```python
from build123d import *

# Parameters (mm, degrees)
SKETCH1_W                = 25
SKETCH1_H                = 25
SKETCH1_W_2              = 21
SKETCH1_H_2              = 21
BOSS_EXTRUDE1_DEPTH      = 200
SKETCH2_W                = 40
SKETCH2_H                = 12
CUT_EXTRUDE1_DEPTH       = 26
SKETCH3_R                = 5
CUT_EXTRUDE2_DEPTH       = 26
BOSS_EXTRUDE2_START      = -40
SKETCH5_W                = 21
SKETCH5_H                = 21
BOSS_EXTRUDE2_DEPTH      = 1
BOSS_EXTRUDE2_DEPTH_BACK = 199
SKETCH3_2_R              = 5
CUT_EXTRUDE4_DEPTH       = 239
SKETCH6_W                = 21
SKETCH6_H                = 12
CUT_EXTRUDE5_DEPTH       = 39
SKETCH8_W                = 21
SKETCH8_H                = 12
BOSS_EXTRUDE3_DEPTH      = 40
SKETCH9_R                = 5
CUT_EXTRUDE6_DEPTH       = 19.5


with BuildPart() as part:
    # Sketch1 → Boss-Extrude1 (new body)
    with BuildSketch(Plane.XY):
        Rectangle(SKETCH1_W, SKETCH1_H)
        Rectangle(SKETCH1_W_2, SKETCH1_H_2, mode=Mode.SUBTRACT)
    extrude(amount=BOSS_EXTRUDE1_DEPTH)

    # Sketch2 → Cut-Extrude1 (cut, through all)
    with BuildSketch(Plane(origin=(12.5, 0, 0), x_dir=(0, 0, -1), z_dir=(1, 0, 0))):
        with Locations((-20, 0)):
            Rectangle(SKETCH2_W, SKETCH2_H)
    extrude(amount=-CUT_EXTRUDE1_DEPTH, mode=Mode.SUBTRACT)

    # Sketch3 → Cut-Extrude2 (cut, through all)
    with BuildSketch(Plane(origin=(0, 12.5, 0), x_dir=(1, 0, 0), z_dir=(0, 1, 0))):
        with Locations((0, -9)):
            Circle(SKETCH3_R)
    extrude(amount=-CUT_EXTRUDE2_DEPTH, mode=Mode.SUBTRACT)

    # Sketch5 → Boss-Extrude2 (add, two sides)
    with BuildSketch(Plane.XY.offset(240).offset(BOSS_EXTRUDE2_START)) as boss_extrude2_sk:
        Rectangle(SKETCH5_W, SKETCH5_H)
    extrude(amount=BOSS_EXTRUDE2_DEPTH)
    extrude(boss_extrude2_sk.sketch, amount=-BOSS_EXTRUDE2_DEPTH_BACK)

    # Sketch3<2> → Cut-Extrude4 (cut)
    with BuildSketch(Plane(origin=(0, 12.5, 0), x_dir=(1, 0, 0), z_dir=(0, 1, 0))):
        with Locations((0, -9)):
            Circle(SKETCH3_2_R)
    extrude(amount=-CUT_EXTRUDE4_DEPTH, mode=Mode.SUBTRACT)

    # Sketch6 → Cut-Extrude5 (cut)
    with BuildSketch(Plane(origin=(0, 0, 1), x_dir=(-1, 0, 0), z_dir=(0, 0, -1))):
        Rectangle(SKETCH6_W, SKETCH6_H)
    extrude(amount=-CUT_EXTRUDE5_DEPTH, mode=Mode.SUBTRACT)

    # Sketch8 → Boss-Extrude3 (add)
    with BuildSketch(Plane.XY.offset(200)):
        Rectangle(SKETCH8_W, SKETCH8_H)
    extrude(amount=BOSS_EXTRUDE3_DEPTH)

    # Sketch9 → Cut-Extrude6 (cut, through all)
    with BuildSketch(Plane(origin=(0, 6, 0), x_dir=(1, 0, 0), z_dir=(0, 1, 0))):
        with Locations((0, -222)):
            Circle(SKETCH9_R)
    extrude(amount=-CUT_EXTRUDE6_DEPTH, mode=Mode.SUBTRACT)


solid = part.part
```
Verification items for the finished model (mm, model axes). A direction names the side the tool comes from. Coordinates: 2 decimals unless noted, no trailing zeros. Order: outer loops, then holes, each group sorted by start corner. A loop starts at its lowest first (then second) coordinate and runs counter-clockwise, first axis right, second up. Notation, with made-up numbers: (48, 1) -> (72, 1) arc R19 cw to (72, 8) -> close; hole circle Ø6 at (44, -36.75). An arc over 180 degrees is marked (long way). Answer as CSV lines item,"result". Start each with the question number.
1) Set-up check for faces 4 (the face through (-10.5, 0, 220)), 5 (the face through (0, 8, 1)), 6 (the face through (0, 6, 216)), 7 (the face through (0, -6, 216)), 8 (the face through (10.5, 0, 220)): record each of +Z, -Z, +X, -X, +Y, -Y from which the full face is reachable in a straight line by a thin tool's end or side.
2) Gauge pin test, flat ends, axial feed: pin 1 Ø1.5 at (x, y) = (3, 5.5) entering from -Z; pin 2 Ø6.5 at (y, z) = (1.5, 212) entering from -X; pin 3 Ø1 at (x, y) = (0, 10) entering from +Z. Record the tip position at first contact, or that the pin passes through.
3) Cross-section at D-D, the plane y = 1.75. Record the boundary of the cut face in (x, z), then the cut area to 3 significant figures.
4) Cross-section at A-A, the plane z = 9. Record the boundary of the cut face in (x, y).
5) Material ranges on L1, parallel to Z at x = 0, y = -3; L2, parallel to Z at x = 0, y = 9.75; L3, parallel to Y at x = 6, z = 28, recorded low to high. Write a range as [from, to].
6) Release check for a two-part mould opening along Y. For faces 1 (the face through (0, -11, 0)), 2 (the face through (0, -12.5, 99)), 3 (the face through (0, 6, 20)) record: released by +Y, released by -Y, zero draft, split by the parting line, or undercut.
7) Cross-section at C-C, the plane z = 222. Record the boundary of the cut face in (x, y).
8) Cross-section at B-B, the plane x = 0. Give the number of separate pieces and of enclosed holes in the cut face, then the cut area to 3 significant figures.
Conclusion:
1,face 4,"+Z, -X, +Y, -Y"
1,face 5,"-Z"
1,face 6,"+Z, +X, -X, +Y"
1,face 7,"+Z, +X, -X, -Y"
1,face 8,"+Z, +X, +Y, -Y"
2,pin 1,"stops at z = 1"
2,pin 2,"stops at x = -10.5"
2,pin 3,"stops at z = 201"
3,outline,"(-12.5, 40) -> (12.5, 40) -> (12.5, 200) -> (10.5, 200) -> (10.5, 240) -> (-10.5, 240) -> (-10.5, 200) -> (-12.5, 200) -> close; hole circle Ø10 at (0, 222)"
3,area,"4,760 mm²"
4,outline,"(-12.5, -12.5) -> (-5, -12.5) -> (-5, -6) -> (-12.5, -6) -> close; (-12.5, 6) -> (-5, 6) -> (-5, 12.5) -> (-12.5, 12.5) -> close; (5, -12.5) -> (12.5, -12.5) -> (12.5, -6) -> (5, -6) -> close; (5, 6) -> (12.5, 6) -> (12.5, 12.5) -> (5, 12.5) -> close"
5,L1,"z = [40, 217], [227, 240]"
5,L2,"z = [1, 4], [14, 201]"
5,L3,"y = [-12.5, -6], [6, 12.5]"
6,face 1,"zero draft"
6,face 2,"released by -Y"
6,face 3,"undercut"
7,outline,"(-10.5, -6) -> (-5, -6) -> (-5, 6) -> (-10.5, 6) -> close; (5, -6) -> (10.5, -6) -> (10.5, 6) -> (5, 6) -> close"
8,separate pieces,"4"
8,enclosed holes,"0"
8,area,"4,750 mm²"
